Part print with two shaded views. Sizes in mm from the minimum x, y, z corner. A direction names the side the tool comes from. Round coordinates to 2 decimals unless told otherwise and drop trailing zeros. Order: outer loops, then holes, each group sorted by start corner. A loop starts at its lowest first (then second) coordinate and runs counter-clockwise, first axis right, second up. Notation, with made-up numbers: (17.5, 14.5) -> (69.5, 14.5) arc R14 cw to (69.5, 38.5) -> close; hole circle Ø9 at (-30.75, 18). An arc over 180 degrees is marked (long way). Answer as a JSON object with one key per item and string values.
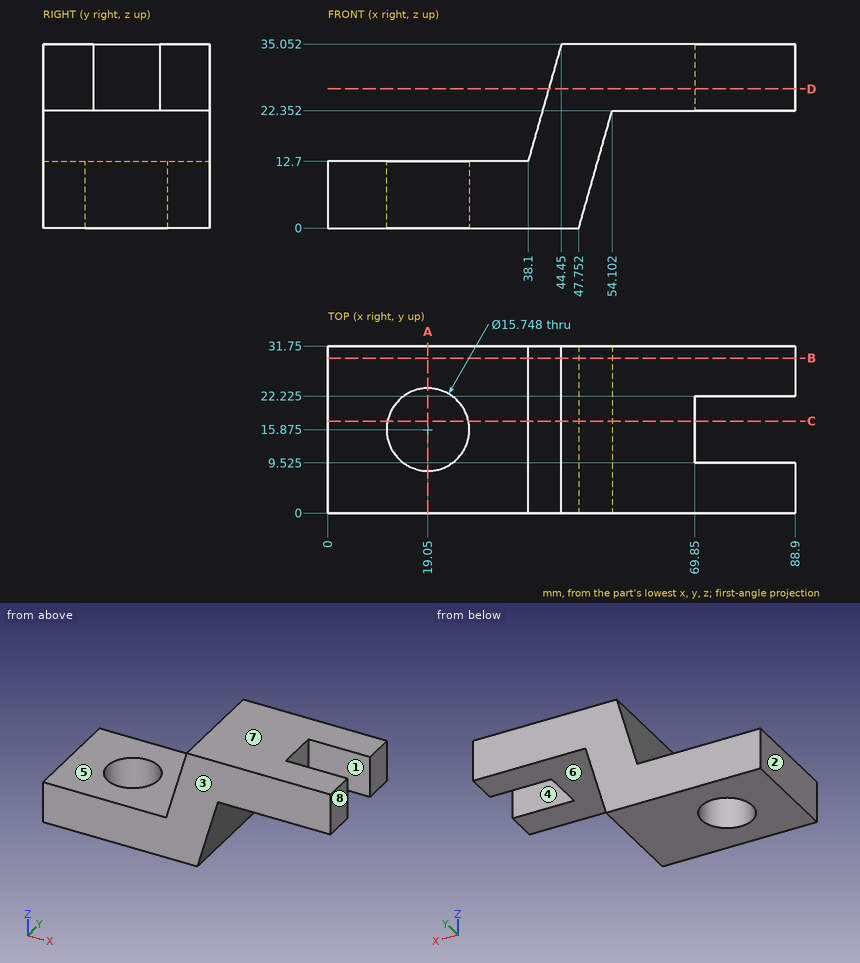
1) Flat gauge pins, fed straight in: pin 1 Ø2 at (x, y) = (64.5, 4.5) entering from -Z; pin 2 Ø4 at (y, z) = (18, 26) entering from +X; pin 3 Ø1 at (y, z) = (10, 11.5) entering from +X. Where does each tip first touch, or does it go through?
Checked values:
{"pin 1": "stops at z = 22.35", "pin 2": "stops at x = 69.85", "pin 3": "stops at x = 51.16"}
2) Cut at C-C, the plane y = 17.5. Give the cut face in (x, z), plus the area to 3 significant figures.
Checked values:
{"outline": "(0, 0) -> (11.35, 0) -> (11.35, 12.7) -> (0, 12.7) -> close; (26.75, 0) -> (47.75, 0) -> (54.1, 22.35) -> (69.85, 22.35) -> (69.85, 35.05) -> (44.45, 35.05) -> (38.1, 12.7) -> (26.75, 12.7) -> close", "area": "907 mm²"}
3) Pull direction Y, two halves, no side cores. Call the marked faces 1, 2 and 3: pulls with the +Y half, pulls with the -Y half, needs draft (parallel to the pull), parting line crosses it, or undercut.
Checked values:
{"face 1": "undercut", "face 2": "needs draft", "face 3": "pulls with the -Y half"}
4) Which spindle directions (+Z, -Z, +X, -X, +Y, -Y) get a long thin tool onto all of the face, cutting with end or side? Do the marked faces 4, 5, 6, 7 and 8. Say none if no direction does.
Checked values:
{"face 4": "+Z, -Z, +X", "face 5": "+Z, -X, +Y, -Y", "face 6": "-Z, +X, +Y, -Y", "face 7": "+Z, +X, -X, +Y, -Y", "face 8": "+Z, -Z, +X, +Y, -Y"}
5) Probe L1, parallel to Y at x = 19, z = 8; L2, parallel to Z at x = 33, y = 23.5; L3, parallel to Z at x = 60.5, y = 20. List the from-to ranges inside material, lowest first. Write a range as from..to.
Checked values:
{"L1": "y = 0..8, 23.75..31.75", "L2": "z = 0..12.7", "L3": "z = 22.35..35.05"}
6) Cut at B-B, the plane y = 29.5. Give the cut face in (x, z), plus the area to 3 significant figures.
Checked values:
{"outline": "(0, 0) -> (47.75, 0) -> (54.1, 22.35) -> (88.9, 22.35) -> (88.9, 35.05) -> (44.45, 35.05) -> (38.1, 12.7) -> (0, 12.7) -> close", "area": "1,340 mm²"}
7) Cut at A-A, the plane x = 19.05. Give the cut face in (y, z), plus the area to 3 significant figures.
Checked values:
{"outline": "(0, 0) -> (8, 0) -> (8, 12.7) -> (0, 12.7) -> close; (23.75, 0) -> (31.75, 0) -> (31.75, 12.7) -> (23.75, 12.7) -> close", "area": "203 mm²"}
8) Cut at D-D, the plane z = 26.5. Give the cut face in (x, y) (3 decimals), plus the area to 3 significant figures.
Checked values:
{"outline": "(42.02, 0) -> (88.9, 0) -> (88.9, 9.525) -> (69.85, 9.525) -> (69.85, 22.225) -> (88.9, 22.225) -> (88.9, 31.75) -> (42.02, 31.75) -> close", "area": "1,250 mm²"}
